from build123d import *

# Parameters (mm, degrees)
SKETCH1_W           = 56
SKETCH1_H           = 56
BOSS_EXTRUDE1_DEPTH = 10.5
SKETCH4_R           = 19
BOSS_EXTRUDE4_DEPTH = 1.5
FILLET1_R           = 0.5
FILLET2_R           = 3
SKETCH5_R           = 6
CUT_EXTRUDE1_DEPTH  = 42.376321731
SKETCH8_W           = 7
SKETCH8_H           = 6
CUT_EXTRUDE2_DEPTH  = 2.7
CIRPATTERN7_COUNT   = 4
FILLET5_R           = 1
FILLET6_R           = 3.5
SKETCH10_W          = 9
SKETCH10_H          = 9
CUT_EXTRUDE4_DEPTH  = 5
CIRPATTERN11_COUNT  = 4
FILLET8_R           = 2
FILLET9_R           = 5
CIRPATTERN12_COUNT  = 4


with BuildPart() as part:
    # Sketch1 → Boss-Extrude1 (new body)
    with BuildSketch(Plane.XY):
        Rectangle(SKETCH1_W, SKETCH1_H)
    extrude(amount=BOSS_EXTRUDE1_DEPTH)

    # Sketch4 → Boss-Extrude4 (add)
    with BuildSketch(Plane(origin=(0, 0, 0), x_dir=(-1, 0, 0), z_dir=(0, 0, -1))):
        with Locations(Location((0, 0, 0), (0, 0, 180))):
            Circle(SKETCH4_R)
    extrude(amount=BOSS_EXTRUDE4_DEPTH)

    # Fillet1
    fillet1_edges = [part.edges().sort_by_distance(p)[0] for p in [
        (-19, 0, 0),
    ]]
    fillet(fillet1_edges, radius=FILLET1_R)

    # Fillet2
    fillet2_edges = [part.edges().sort_by_distance(p)[0] for p in [
        (-28, 28, 5.25),
        (28, 28, 5.25),
        (28, -28, 5.25),
        (-28, -28, 5.25),
    ]]
    fillet(fillet2_edges, radius=FILLET2_R)

    # Sketch5 → Cut-Extrude1 (cut, through all)
    with BuildSketch(Plane(origin=(0, 0, -1.5), x_dir=(-1, 0, 0), z_dir=(0, 0, -1))):
        Circle(SKETCH5_R)
    extrude(amount=-CUT_EXTRUDE1_DEPTH, mode=Mode.SUBTRACT)

    # Sketch7 → Ø5.0mm Dowel Hole1 (revolve, cut)
    with BuildSketch(Plane(origin=(23.5, 23.5, 0), x_dir=(0, 1, 0), z_dir=(1, 0, 0))):
        Polygon((0, 0), (0, 18.502151548), (2.5, 17), (2.5, 0), align=None)
    f_5_0mm_dowel_hole1 = revolve(axis=Axis((23.5, 23.5, -6.35), (0, 0, 1)), mode=Mode.SUBTRACT)

    # Sketch8 → Cut-Extrude2 (cut)
    with BuildSketch(Plane(origin=(0, 0, 0), x_dir=(-1, 0, 0), z_dir=(0, 0, -1))):
        with Locations((15.5, 25)):
            Rectangle(SKETCH8_W, SKETCH8_H)
    cut_extrude2 = extrude(amount=-CUT_EXTRUDE2_DEPTH, mode=Mode.SUBTRACT)

    # CirPattern7: Cut-Extrude2 ×4 about axis
    cirpattern7_axis = Axis((0, 0, 0), (0, 0, 1))
    for i in range(1, CIRPATTERN7_COUNT):
        add(cut_extrude2.rotate(cirpattern7_axis, i * 360 / CIRPATTERN7_COUNT), mode=Mode.SUBTRACT)

    # Fillet5
    fillet5_edges = [part.edges().sort_by_distance(p)[0] for p in [
        (-28, -12, 1.35),
        (-28, -19, 1.35),
        (-12, 28, 1.35),
        (-19, 28, 1.35),
        (28, 12, 1.35),
        (28, 19, 1.35),
        (12, -28, 1.35),
        (19, -28, 1.35),
    ]]
    fillet(fillet5_edges, radius=FILLET5_R)

    # Fillet6
    fillet6_edges = [part.edges().sort_by_distance(p)[0] for p in [
        (-12, 22, 1.35),
        (-19, 22, 1.35),
        (22, 12, 1.35),
        (22, 19, 1.35),
        (12, -22, 1.35),
        (19, -22, 1.35),
        (-22, -19, 1.35),
        (-22, -12, 1.35),
    ]]
    fillet(fillet6_edges, radius=FILLET6_R - 0.0001)  # a hair under: the kernel refuses the full size

    # Sketch10 → Cut-Extrude4 (cut)
    with BuildSketch(Plane.XY.offset(10.5)):
        with Locations((-23.5, 23.5)):
            Rectangle(SKETCH10_W, SKETCH10_H)
    cut_extrude4 = extrude(amount=-CUT_EXTRUDE4_DEPTH, mode=Mode.SUBTRACT)

    # CirPattern11: Cut-Extrude4 ×4 about axis
    cirpattern11_axis = Axis((0, 0, 0), (0, 0, 1))
    for i in range(1, CIRPATTERN11_COUNT):
        add(cut_extrude4.rotate(cirpattern11_axis, i * 360 / CIRPATTERN11_COUNT), mode=Mode.SUBTRACT)

    # Fillet8
    fillet8_edges = [part.edges().sort_by_distance(p)[0] for p in [
        (-28, 19, 8),
        (-19, 28, 8),
        (19, 28, 8),
        (28, 19, 8),
        (28, -19, 8),
        (19, -28, 8),
        (-19, -28, 8),
        (-28, -19, 8),
    ]]
    fillet(fillet8_edges, radius=FILLET8_R)

    # Fillet9
    fillet9_edges = [part.edges().sort_by_distance(p)[0] for p in [
        (-19, 19, 8),
        (19, 19, 8),
        (19, -19, 8),
        (-19, -19, 8),
    ]]
    fillet(fillet9_edges, radius=FILLET9_R)

    # CirPattern12: Ø5.0mm Dowel Hole1 ×4 about axis
    cirpattern12_axis = Axis((0, 0, 0), (0, 0, 1))
    for i in range(1, CIRPATTERN12_COUNT):
        add(f_5_0mm_dowel_hole1.rotate(cirpattern12_axis, i * 360 / CIRPATTERN12_COUNT), mode=Mode.SUBTRACT)


solid = part.part
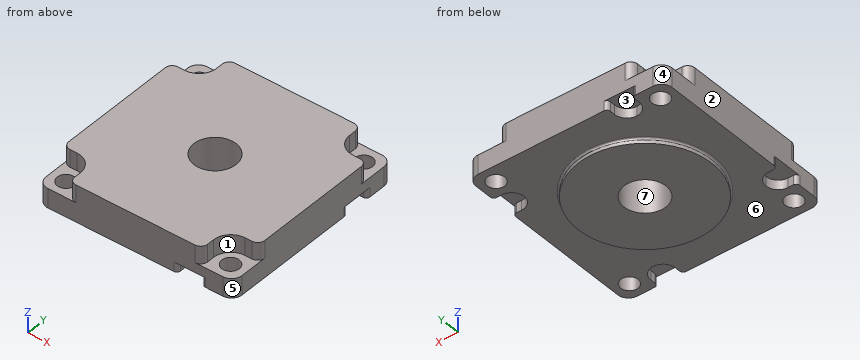
For this review, take the finished solid that the model builds, in its own axes (mm). Face numbers are marked on the shaded views. A direction names the side the tool comes from. Give positions to 0.01 mm unless a question says otherwise; leave off trailing zeros. Loops run counter-clockwise (first coordinate to the right, second up) from the corner with the lowest first, then second, coordinate; pieces in that order, holes last. Notation, with made-up numbers: M 73,39.5 L 107,39.5 A16 cw 107,54.5 Z; hole C 79.25,60 d11. An arc over 180 degrees is marked long. Answer as a JSON object with one key per item and string values. Group by question number.
Q1. For probe 1 along Y at (x, z) = (-23.5, 3.7); probe 2 along Y at (x, z) = (-21.5, 5), list the stretches that pass through material, from the lowest coordinate up. Write a range as [from, to].
Q2. Tool access review of the marked faces 1, 2 and 3: name each direction out of +Z, -Z, +X, -X, +Y, -Y from which nothing blocks a thin tool from reaching the whole face with its end or side.
Q3. Add section D-D on z = 9.75. Give the boundary of the cut face in (x, y), and give its area (3 significant figures).
Q4. Insertion check: P1, Ø2, axis at y = -24.5, z = 8, coming from the -X side; P2, Ø1.8, axis at x = 26, y = 15.5, coming from the -Z side; P3, Ø3, axis at x = 23.5, y = -23.5, coming from the -Z side; P4, Ø6, axis at x = 20, y = 18.5, coming from the -Z side. Each pin has a flat end and moves straight along its axis. Give the tip position at first contact, or say it passes through.
Q5. Add section B-B on x = 0. Give the boundary of the cut face in (y, z).
Q6. Mouldability with a two-part tool opening along Y and no side actions: class the marked faces 4, 5, 6 and 7 as +Y half, -Y half, draft (parallel to the pull), parting line (faces both ways), or undercut.
Q7. Add section A-A on z = 4.5. Give the boundary of the cut face in (x, y).
Checked values:
{
 "1": {"probe 1": "[-28, -26], [-21, 21], [26, 28]", "probe 2": "[-28, -25], [-22, 22], [25, 28]"},
 "2": {"face 1": "+Z, +X, -Y", "face 2": "+Z, -Z, -X, +Y, -Y", "face 3": "-Z, +Y"},
 "3": {"outline": "M -28,-17 A2 ccw -26,-19 L -24,-19 A5 cw -19,-24 L -19,-26 A2 ccw -17,-28 L 17,-28 A2 ccw 19,-26 L 19,-24 A5 cw 24,-19 L 26,-19 A2 ccw 28,-17 L 28,17 A2 ccw 26,19 L 24,19 A5 cw 19,24 L 19,26 A2 ccw 17,28 L -17,28 A2 ccw -19,26 L -19,24 A5 cw -24,19 L -26,19 A2 ccw -28,17 Z; hole C 0,0 d12", "area": "2,710 mm²"},
 "4": {"P1": "x = -19.03", "P2": "z = 2.7", "P3": "through", "P4": "z = 0"},
 "5": {"outline": "M -28,0 L -19.5,0 A0.5 cw -19,-0.5 L -19,-1.5 L -6,-1.5 L -6,10.5 L -28,10.5 Z; M 6,-1.5 L 19,-1.5 L 19,-0.5 A0.5 cw 19.5,0 L 28,0 L 28,10.5 L 6,10.5 Z"},
 "6": {"face 4": "+Y half", "face 5": "-Y half", "face 6": "draft", "face 7": "undercut"},
 "7": {"outline": "M -28,-25 A3 ccw -25,-28 L 25,-28 A3 ccw 28,-25 L 28,25 A3 ccw 25,28 L -25,28 A3 ccw -28,25 Z; hole C -23.5,-23.5 d5; hole C -23.5,23.5 d5; hole C 0,0 d12; hole C 23.5,-23.5 d5; hole C 23.5,23.5 d5"}
}
